Here's how the part is built. I have some questions about the finished solid (model axes, mm). A direction names the side the tool comes from. Give positions to 0.01 mm unless a question says otherwise; leave off trailing zeros. Loops run counter-clockwise (first coordinate to the right, second up) from the corner with the lowest first, then second, coordinate; pieces in that order, holes last. Notation, with made-up numbers: (61, -22) - (90, -22) arc R28 ccw to (90, 16) - close; hole circle Ø3 at (72.5, 13.25). An arc over 180 degrees is marked (long way). Use a Markdown table: item, result.
from build123d import *

# Parameters (mm, degrees)
CUT_EXTRUDE1_DEPTH      = 20.05
CUT_EXTRUDE1_DEPTH_BACK = 20.05
FILLET1_R               = 2.54
CHAMFER1_SIZE           = 1.27


with BuildPart() as part:
    # Sketch1 → Revolve1 (revolve)
    with BuildSketch(Plane(origin=(0, 0, 0), x_dir=(1, 0, 0), z_dir=(0, 1, 0))):
        Polygon((12.7, 0), (15.875, 0), (15.875, 6.35), (19.05, 6.35), (19.05, 12.7), (0, 12.7), (0, 6.35), (12.7, 6.35), align=None)
    revolve(axis=Axis((0, 0, 31.989022308), (0, 0, -1)))

    # Sketch2 → Cut-Extrude1 (cut, two sides)
    with BuildSketch(Plane(origin=(0, 0, 0), x_dir=(0, 0, -1), z_dir=(1, 0, 0))) as cut_extrude1_sk:
        Polygon((71.164271634, -1.5875), (12.7, -1.5875), (9.525, -1.5875), (9.525, 1.5875), (12.7, 1.5875), (71.164271634, 1.5875), (188.092814902, 1.5875), (188.092814902, -1.5875), align=None)
    extrude(amount=CUT_EXTRUDE1_DEPTH, mode=Mode.SUBTRACT)
    extrude(cut_extrude1_sk.sketch, amount=-CUT_EXTRUDE1_DEPTH_BACK, mode=Mode.SUBTRACT)

    # Fillet1
    fillet1_edges = [part.edges().sort_by_distance(p)[0] for p in [
        (0, -19.05, -12.7),
        (0, 19.05, -12.7),
    ]]
    fillet(fillet1_edges, radius=FILLET1_R)

    # Chamfer1
    chamfer1_edges = [part.edges().sort_by_distance(p)[0] for p in [
        (-15.875, 0, 0),
    ]]
    chamfer(chamfer1_edges, length=CHAMFER1_SIZE)


solid = part.part
(1) Suppose I cut it at D-D on z = -7. Write out the boundary of the cut face in (x, y).
A:
| item | result |
|---|---|
| outline | circle Ø38.1 at (0, 0) |
(2) Will these pins go through, and if not, where does the flat tip stop? pin 1 (1.5 mm diameter, centred on x = 4, y = -8, fed in from +Z); pin 2 (1.6 mm diameter, centred on x = 8.5, z = -11, fed in from -Y); pin 3 (3.5 mm diameter, centred on x = -2.5, y = 0.5, fed in from -Z); pin 4 (2 mm diameter, centred on y = -13, z = -8.5, fed in from -X).
A:
| item | result |
|---|---|
| pin 1 | z = -6.35 |
| pin 2 | y = -17.34 |
| pin 3 | z = -12.7 |
| pin 4 | x = -14.8 |
(3) Suppose I cut it at C-C on z = -4.25. Write out the boundary of the cut face in (x, y) (3 decimals), plus the area to 3 significant figures.
A:
| item | result |
|---|---|
| outline | circle Ø31.75 at (0, 0); hole circle Ø25.4 at (0, 0) |
| area | 285 mm2 |
(4) If I drill on line 1 (Y direction, x = 0, z = -1.5) (3 decimals); line 2 (Z direction, x = 7.5, y = 5), over which ranges is the centre line in solid material (lowest first)?
A:
| item | result |
|---|---|
| line 1 | -15.875 to -12.7, 12.7 to 15.875 |
| line 2 | -12.7 to -6.35 |
(5) We'd pull the mould along Y, two halves only. Please class faces 4 (the face through (-2.75, 12.4, -3.13)), 5 (the face through (18.17, -5.72, -8.28)), 6 (the face through (4, -16, -6.35)), 7 (the face through (0, 0, -9.525)): pulls with the +Y half, pulls with the -Y half, needs draft (parallel to the pull), parting line crosses it, or undercut.
A:
| item | result |
|---|---|
| face 4 | undercut |
| face 5 | parting line crosses it |
| face 6 | needs draft |
| face 7 | undercut |
(6) Suppose I cut it at A-A on y = 0. Write out the boundary of the cut face in (x, z) (3 decimals).
A:
| item | result |
|---|---|
| outline | (-19.05, -9.525) - (19.05, -9.525) - (19.05, -6.35) - (15.875, -6.35) - (15.875, -1.27) - (14.605, 0) - (12.7, 0) - (12.7, -6.35) - (-12.7, -6.35) - (-12.7, 0) - (-14.605, 0) - (-15.875, -1.27) - (-15.875, -6.35) - (-19.05, -6.35) - close |
(7) On a 3-axis mill with a long thin cutter (end or side, diameter ignored), from which of +Z, -Z, +X, -X, +Y, -Y can I reach the whole of each face in a straight line? I mean faces 1 (the face through (-3.441, 15.497, -3.846)), 2 (the face through (0, -1.588, -11)), 3 (the face through (0, -7, -12.7)). Say none if no direction works.
A:
| item | result |
|---|---|
| face 1 | +Z |
| face 2 | -Z, +X, -X |
| face 3 | -Z, +X, -X, +Y, -Y |
